from build123d import *

# Parameters (mm, degrees)
BOSS_EXTRUDE1_DEPTH = 10
BOSS_EXTRUDE2_DEPTH = 10
BOSS_EXTRUDE3_DEPTH = 10


with BuildPart() as part:
    # Sketch20 → Boss-Extrude1 (new body)
    with BuildSketch(Plane.XY):
        Polygon((-2.790049513, 109.432186673), (-1.434483855, -10.567813327), (55.586408616, 16.767282175), (53.501321505, 49.432186673), (52.169506721, 82.106882469), align=None)
    extrude(amount=BOSS_EXTRUDE1_DEPTH)

    # Sketch21 → Boss-Extrude2 (add)
    with BuildSketch(Plane(origin=(0, 0, 0), x_dir=(-1, 0, 0), z_dir=(0, 0, -1))):
        Polygon((2.153425382, 53.075716438), (-6.504020667, 53.075716438), (-6.504020667, 44.793833992), (2.059870087, 44.793833992), align=None)
        Polygon((-53.35281188, 53.075716438), (-44.305813439, 53.075716438), (-44.305813439, 44.793833992), (-53.797399805, 44.793833992), align=None)
        Polygon((-20.609929611, 0), (-20.609929611, 9.183356753), (-28.35805903, 10.939673778), (-28.35805903, 3.714355361), align=None)
        Polygon((-28.35805903, 93.945679874), (-28.35805903, 87.903711829), (-20.609929611, 87.903711829), (-20.609929611, 97.797967044), align=None)
    extrude(amount=BOSS_EXTRUDE2_DEPTH)

    # Sketch22 → Boss-Extrude3 (add)
    with BuildSketch(Plane(origin=(0, 0, -10), x_dir=(-1, 0, 0), z_dir=(0, 0, -1))):
        Polygon((-24.483994321, 1.85717768), (2.707182476, -11.177928968), (3.725282972, 78.948328543), (3.725282972, 110.997079558), (-55.502382997, 81.814284871), (-58.856312716, 16.677185524), align=None)
    extrude(amount=BOSS_EXTRUDE3_DEPTH)


solid = part.part
Read the model definition and answer for the solid it produces. Units are mm, in the model's axes. A direction names the side the tool comes from. Round coordinates to 2 decimals unless told otherwise and drop trailing zeros. Loops run counter-clockwise (first coordinate to the right, second up) from the corner with the lowest first, then second, coordinate; pieces in that order, holes last.
Q1. Consider probe 1 along Z at (x, y) = (18.5, 4.5); probe 2 along Y at (x, z) = (5, -2.5); probe 3 along X at (y, z) = (91.5, -9.5). Determine where each line is inside the solid, lowest interval first.
Q2. Section D-D on z = 5.75 is taken. Write down the section's boundary in (x, y), and give its area (3 significant figures).
Q3. Section A-A on z = -4.5 is taken. Write down the section's boundary in (x, y), and give its area (3 significant figures).
Q4. Section B-B on x = 31.5 is taken. Write down the section's boundary in (y, z), and give its area (3 significant figures).
Q5. Which of the six approach directions +Z, -Z, +X, -X, +Y, -Y give full straight-line access (tool end or side, diameter ignored) to faces 1 (the face through (49, 44.794, -5)), 2 (the face through (54.56, 32.87, 4.93)), 3 (the face through (20, 50, 0))?
Q6. Determine the mould class of faces 4 (the face through (25.47, 96.61, -14.93)), 5 (the face through (2, 53.076, -5)), 6 (the face through (6.504, 49, -5)), 7 (the face through (20.61, 93, -5)) for opening direction X: released by +X, released by -X, zero draft, split by the parting line, or undercut.
Q7. Section C-C on y = 20 is taken. Write down the section's boundary in (x, z).
Q8. Each of these flat-tipped pins is pushed along its axis until it touches: pin 1 (5 mm diameter, centred on y = 91.5, z = -7, fed in from +X); pin 2 (1.5 mm diameter, centred on y = 30, z = -13, fed in from +X); pin 3 (2.5 mm diameter, centred on x = 4, z = -6.5, fed in from +Y); pin 4 (8 mm diameter, centred on y = 93, z = -6.5, fed in from -X). Where does it stop, or does it pass through?
Output:
1. probe 1: z = -20 to -10, 0 to 10
1. probe 2: y = 44.79 to 53.08
1. probe 3: x = 20.61 to 28.36
2. outline: (-2.79, 109.43) - (-1.43, -10.57) - (55.59, 16.77) - (53.5, 49.43) - (52.17, 82.11) - close
2. area: 5,180 mm2
3. outline: (-2.15, 53.08) - (-2.06, 44.79) - (6.5, 44.79) - (6.5, 53.08) - close; (20.61, 0) - (28.36, 3.71) - (28.36, 10.94) - (20.61, 9.18) - close; (20.61, 87.9) - (28.36, 87.9) - (28.36, 93.95) - (20.61, 97.8) - close; (44.31, 44.79) - (53.8, 44.79) - (53.35, 53.08) - (44.31, 53.08) - close
3. area: 273 mm2
4. outline: (4.88, -20) - (93.64, -20) - (93.64, -10) - (4.88, -10) - close; (5.22, 0) - (92.38, 0) - (92.38, 10) - (5.22, 10) - close
4. area: 1,760 mm2
5. face 1: +X, -X, -Y
5. face 2: +Z, +X, +Y
5. face 3: none
6. face 4: released by +X
6. face 5: zero draft
6. face 6: undercut
6. face 7: released by -X
7. outline: (-3.06, -20) - (58.69, -20) - (58.69, -10) - (-3.06, -10) - close; (-1.78, 0) - (55.38, 0) - (55.38, 10) - (-1.78, 10) - close
8. pin 1: stops at x = 28.36
8. pin 2: stops at x = 58.21
8. pin 3: stops at y = 53.08
8. pin 4: stops at x = -3.73
